```python
from build123d import *

# Parameters (mm, degrees)
F2_SIZE2 = 2
F2_SIZE  = 2
F3_R     = 3
F4_SIZE  = 5


with BuildPart() as f1:
    # F0 (on Top) → F1 (revolve)
    with BuildSketch(Plane.XY):
        Polygon((68.342246, 0), (-39.657754, 0), (-39.657754, -11), (-1.657754, -11), (-1.657754, -18), (18.342246, -18), (18.342246, -21), (30.342246, -21), (30.342246, -18), (40.342246, -18), (40.342246, -10), (45.342246, -10), (45.342246, -7), (48.342246, -7), (48.342246, -10), (53.342246, -10), (68.342246, -5), align=None)
    revolve(axis=Axis((14.342246, 0, 0), (1, 0, 0)))

    # F2
    f2_edges = [f1.edges().sort_by_distance(p)[0] for p in [
        (-39.657754, 11, 0),
    ]]
    chamfer(f2_edges, length=F2_SIZE, length2=F2_SIZE2)

    # F3
    f3_edges = [f1.edges().sort_by_distance(p)[0] for p in [
        (-1.657754, 18, 0),
        (-1.657754, 11, 0),
    ]]
    fillet(f3_edges, radius=F3_R)

    # F4
    f4_edges = [f1.edges().sort_by_distance(p)[0] for p in [
        (40.342246, 18, 0),
    ]]
    chamfer(f4_edges, length=F4_SIZE)


solid = f1.part
```
Work out the finished part from the listing and answer in its coordinate system (mm). A direction names the side the tool comes from. Give positions to 0.01 mm unless a question says otherwise; leave off trailing zeros. Write each loop counter-clockwise with the first axis right and the second up, starting at its lowest first coordinate (ties: lowest second). Pieces come first, ordered by that corner, then holes. Notation, with made-up numbers: (-9.5, -24) - (21.5, -24) arc R16 cw to (21.5, -6) - close; hole circle Ø5 at (42, -28). An arc over 180 degrees is marked (long way). Use one line per item in the form item = value.
1. A cutting plane is placed at A-A (x = 8.5). Write down the section's boundary in (y, z), and give its area (3 significant figures).
Filled in:
outline = circle Ø36 at (0, 0)
area = 1,020 mm^2
2. Consider L1, parallel to X at y = -9, z = -18; L2, parallel to X at y = -6, z = 4.5; L3, parallel to X at y = -9, z = 5.5. Determine where each line is inside the solid, lowest interval first.
Filled in:
L1 = 18.34 to 30.34
L2 = -39.66 to 45.34, 48.34 to 60.84
L3 = -38.11 to 40.34
3. Determine the mould class of faces 1 (the face through (46.863, -6.466, 2.681)), 2 (the face through (24.43, -20.03, -6.31)), 3 (the face through (40, 3, 13)) for opening direction X: released by +X, released by -X, zero draft, split by the parting line, or undercut.
Filled in:
face_1 = undercut
face_2 = zero draft
face_3 = released by +X
4. Each of these flat-tipped pins is pushed along its axis until it touches: pin 1 Ø12 at (x, y) = (1.5, -7) entering from +Z; pin 2 Ø10 at (x, y) = (-16, -7) entering from +Z; pin 3 Ø5 at (y, z) = (-5, -16.5) entering from -X. Where does it stop, or does it pass through?
Filled in:
pin_1 = 17.97
pin_2 = 10.82
pin_3 = -1.66
5. For faces 4 (the face through (18.342, -9, -16)), 5 (the face through (30.342, 9, -16)), 6 (the face through (68.342, 0, 0)), 7 (the face through (48.342, 2, -7)), 8 (the face through (-39.658, 0, 0)), determine the directions among +Z, -Z, +X, -X, +Y, -Y from which every point of the face is accessible in a straight line to the end or side of a thin tool.
Filled in:
face_4 = -X
face_5 = +X
face_6 = +Z, -Z, +X, +Y, -Y
face_7 = none
face_8 = +Z, -Z, -X, +Y, -Y
6. A cutting plane is placed at B-B (x = 56.5). Write down the section's boundary in (y, z).
Filled in:
outline = circle Ø17.89 at (0, 0)
